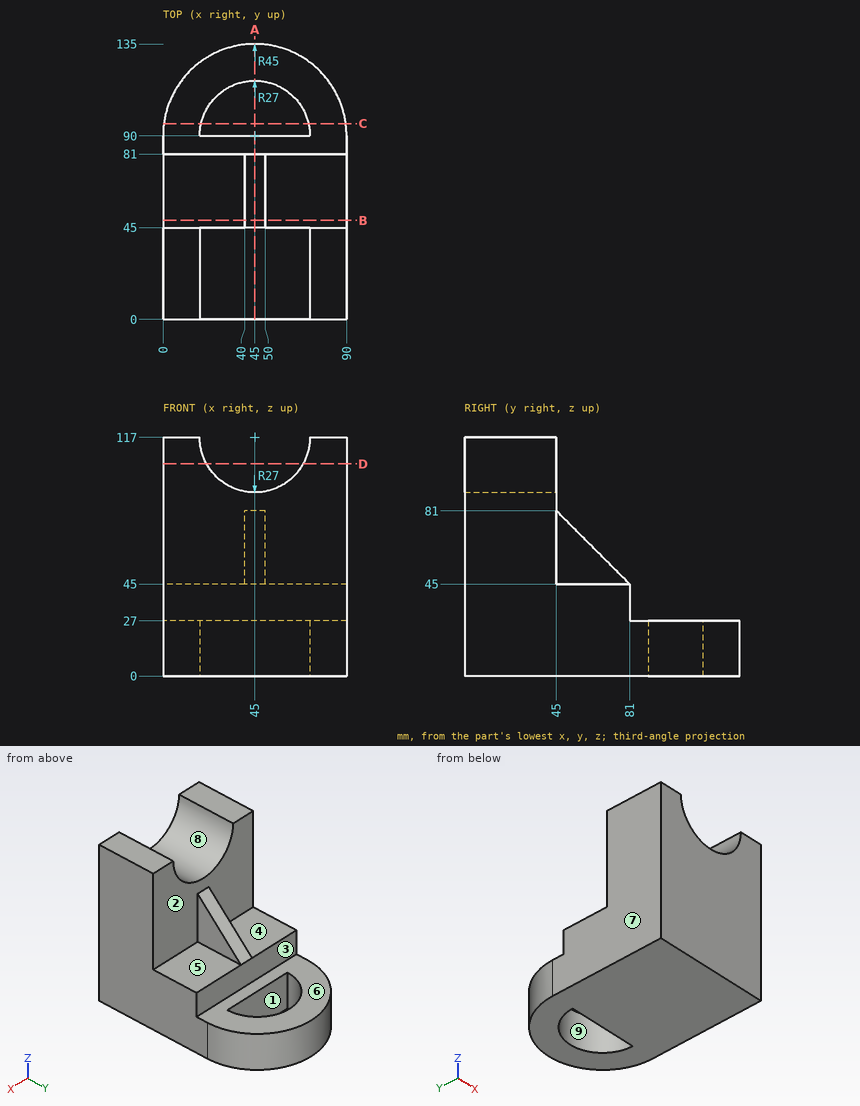
The figure shows three views and two pictorial views of one solid part (mm, origin at its lowest corner). Answer the questions. A direction names the side the tool comes from. Give positions to 0.01 mm unless a question says otherwise; leave off trailing zeros. Order: outer loops, then holes, each group sorted by start corner. A loop starts at its lowest first (then second) coordinate and runs counter-clockwise, first axis right, second up. Notation, with made-up numbers: (-18, -31.5) -> (16, -31.5) arc R23 cw to (16, -3.5) -> close; hole circle Ø7 at (24.5, 67.5). An arc over 180 degrees is marked (long way). One line per item, written item: value.
1) Find section C-C, the plane y = 96. Determine the outline of the cut face in (x, z), plus the area to 3 significant figures.
Reported:
outline: (0.4, 0) -> (18.68, 0) -> (18.68, 27) -> (0.4, 27) -> close; (71.32, 0) -> (89.6, 0) -> (89.6, 27) -> (71.32, 27) -> close
area: 987 mm^2
2) A tool of negligible diameter and unlimited length cuts with its end or side. For the marked faces 1, 2, 3, 4 and 5, from which of +Z, -Z, +X, -X, +Y, -Y can it reach the whole face along a straight path? Write none if from no direction.
Reported:
face 1: +Z, -Z
face 2: +Z, +Y
face 3: +Z, +X, -X, +Y
face 4: +Z, -X, +Y
face 5: +Z, +X, +Y
3) Determine the mould class of the marked faces 6, 7, 8 and 9 for opening direction X: pulls with the +X half, pulls with the -X half, needs draft (parallel to the pull), parting line crosses it, or undercut.
Reported:
face 6: needs draft
face 7: pulls with the -X half
face 8: undercut
face 9: undercut
4) Find section A-A, the plane x = 45. Determine the outline of the cut face in (y, z).
Reported:
outline: (0, 0) -> (90, 0) -> (90, 27) -> (81, 27) -> (81, 45) -> (45, 81) -> (45, 90) -> (0, 90) -> close; (117, 0) -> (135, 0) -> (135, 27) -> (117, 27) -> close
5) Flat-ended cylindrical pins translate along their axes: P1, Ø12, axis at x = 56.5, y = 47, coming from the -Z side; P2, Ø11, axis at x = 28.5, y = 68.5, coming from the +Z side; P3, Ø3, axis at x = 34, z = 35, coming from the +Y side; P4, Ø12, axis at x = 75, z = 99.5, coming from the +Y side. Find the tip coordinate at first contact, or state that the pin passes through.
Reported:
P1: stops at z = 0
P2: stops at z = 45
P3: stops at y = 81
P4: stops at y = 45
6) Find section B-B, the plane y = 48.5. Determine the outline of the cut face in (x, z).
Reported:
outline: (0, 0) -> (90, 0) -> (90, 45) -> (50, 45) -> (50, 77.5) -> (40, 77.5) -> (40, 45) -> (0, 45) -> close
7) Find section D-D, the plane z = 104. Determine the outline of the cut face in (x, y).
Reported:
outline: (0, 0) -> (21.34, 0) -> (21.34, 45) -> (0, 45) -> close; (68.66, 0) -> (90, 0) -> (90, 45) -> (68.66, 45) -> close
8) Find the intervals of material crossed by line 1 (Z direction, x = 78, y = 94.5); line 2 (Z direction, x = 60, y = 58), in increasing order.
Reported:
line 1: z = 0 to 27
line 2: z = 0 to 45
